Can you work these out from the model? Positions are in its coordinate system, mm. Face numbers are marked on the shaded views. A direction names the side the tool comes from. Coordinates: 2 decimals unless noted, no trailing zeros. Order: outer loops, then holes, each group sorted by start corner. A loop starts at its lowest first (then second) coordinate and runs counter-clockwise, first axis right, second up. Notation, with made-up numbers: (27.25, -7.75) -> (44.25, -7.75) arc R23 ccw to (44.25, 1.25) -> close; hole circle Ø6 at (56, 7.25). An arc over 180 degrees is marked (long way). Answer in a Markdown table with one row per item. Add a question column.
1. Imagine slicing it at D-D on y = -4.25. Write out the boundary of the cut face in (x, z), plus the area to 3 significant figures.
2. We'd pull the mould along Y, two halves only. Please class the marked faces 1, 2 and 3: pulls with the +Y half, pulls with the -Y half, needs draft (parallel to the pull), parting line crosses it, or undercut.
3. Will these pins go through, and if not, where does the flat tip stop? pin 1 (5 mm diameter, centred on y = -6.5, z = -10.5, fed in from +X); pin 2 (11 mm diameter, centred on y = -1, z = -21.5, fed in from +X); pin 3 (3 mm diameter, centred on y = -2.5, z = -21, fed in from -X); pin 4 (3 mm diameter, centred on x = 6.5, y = 7, fed in from +Z).
4. Imagine slicing it at B-B on x = 0. Write out the boundary of the cut face in (y, z) (1 decimal).
5. Imagine slicing it at A-A on y = 0. Write out the boundary of the cut face in (x, z) (3 decimals), plus the area to 3 significant figures.
6. If I drill on line 1 along Y through (x, z) = (0.25, -11.5); line 2 along Z through (x, y) = (6.75, 4.25); line 3 along Z through (x, y) = (-7.25, -0.5), over which ranges is the centre line in solid material (lowest first)? Write a range as [from, to].
7. Imagine slicing it at C-C on z = -22. Write out the boundary of the cut face in (x, y).
8. On a 3-axis mill with a long thin cutter (end or side, diameter ignored), from which of +Z, -Z, +X, -X, +Y, -Y can I reach the whole of each face in a straight line? I mean the marked faces 4, 5 and 6. Say none if no direction works.
from build123d import *

# Parameters (mm, degrees)
SKETCH1_R               = 4.725
BOSS_EXTRUDE1_DEPTH     = 12
SKETCH2_R               = 3.46
BOSS_EXTRUDE2_DEPTH     = 15
SKETCH5_R               = 10
BOSS_EXTRUDE3_DEPTH     = 15
CUT_EXTRUDE1_DEPTH      = 5
CUT_EXTRUDE1_DEPTH_BACK = 15
SKETCH4_W               = 2
SKETCH4_H               = 12
CUT_EXTRUDE2_DEPTH      = 10
CUT_EXTRUDE3_REACH      = 35.956
SKETCH6_R               = 2


with BuildPart() as part:
    # Sketch1 → Boss-Extrude1 (new body)
    with BuildSketch(Plane.XY):
        Circle(SKETCH1_R)
    extrude(amount=-BOSS_EXTRUDE1_DEPTH)

    # Sketch2 → Boss-Extrude2 (add)
    with BuildSketch(Plane.XY):
        Circle(SKETCH2_R)
    extrude(amount=BOSS_EXTRUDE2_DEPTH)

    # Sketch5 → Boss-Extrude3 (add)
    with BuildSketch(Plane(origin=(0, 0, -12), x_dir=(-1, 0, 0), z_dir=(0, 0, -1))):
        Circle(SKETCH5_R)
    extrude(amount=BOSS_EXTRUDE3_DEPTH)

    # Sketch3 → Cut-Extrude1 (cut, two sides: drawn at the far end of the back side and taken through both)
    with BuildSketch(Plane(origin=(0, 0, 0), x_dir=(0, 0, -1), z_dir=(1, 0, 0)).offset(-CUT_EXTRUDE1_DEPTH_BACK)):
        Polygon((27, -5), (27, 5), (17, 7.679491924), (17, -7.679491924), align=None)
    extrude(amount=CUT_EXTRUDE1_DEPTH + CUT_EXTRUDE1_DEPTH_BACK, mode=Mode.SUBTRACT)

    # Sketch4 → Cut-Extrude2 (cut)
    with BuildSketch(Plane(origin=(0, 0, -27), x_dir=(-1, 0, 0), z_dir=(0, 0, -1))):
        with Locations((-9, 0)):
            Rectangle(SKETCH4_W, SKETCH4_H)
    extrude(amount=-CUT_EXTRUDE2_DEPTH, mode=Mode.SUBTRACT)

    # Sketch6 → Cut-Extrude3 (cut, up to next)
    with BuildSketch(Plane(origin=(8, 0, 0), x_dir=(0, 0, -1), z_dir=(1, 0, 0)), mode=Mode.PRIVATE) as cut_extrude3_sk1:
        with Locations((22, 0)):
            Circle(SKETCH6_R)
    cut_extrude3_tool1 = extrude(cut_extrude3_sk1.sketch, amount=-CUT_EXTRUDE3_REACH, mode=Mode.PRIVATE) & part.part
    add(cut_extrude3_tool1.solids().sort_by_distance((8, 0, -22))[0], mode=Mode.SUBTRACT)


solid = part.part
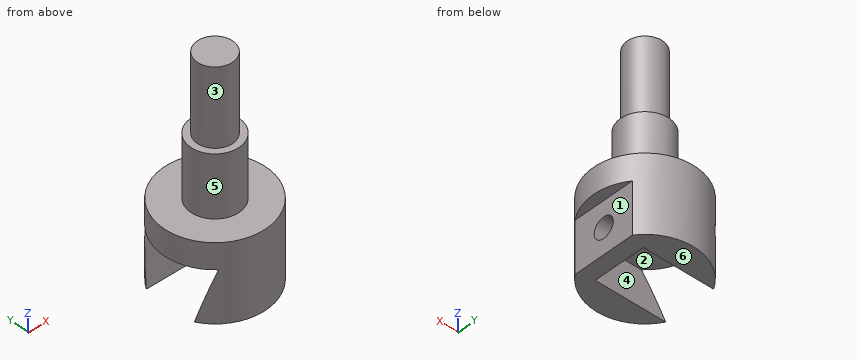
Answers follow:
| question | item | result |
|---|---|---|
| 1 | outline | (-9.05, -17) -> (5, -17) -> (5, -27) -> (8, -27) -> (8, -17) -> (9.05, -17) -> (9.05, -12) -> (2.06, -12) -> (2.06, 0) -> (-2.06, 0) -> (-2.06, -12) -> (-9.05, -12) -> close |
| 1 | area | 170 mm² |
| 2 | face 1 | needs draft |
| 2 | face 2 | undercut |
| 2 | face 3 | parting line crosses it |
| 3 | pin 1 | stops at x = 8.93 |
| 3 | pin 2 | stops at x = 10 |
| 3 | pin 3 | stops at x = 5 |
| 3 | pin 4 | stops at z = -12 |
| 4 | outline | (-10, -27) -> (-5, -27) -> (-7.7, -17) -> (7.7, -17) -> (5, -27) -> (10, -27) -> (10, -12) -> (4.7, -12) -> (4.7, 0) -> (3.5, 0) -> (3.5, 15) -> (-3.5, 15) -> (-3.5, 0) -> (-4.7, 0) -> (-4.7, -12) -> (-10, -12) -> close |
| 5 | outline | (-10, -17) -> (5, -17) -> (5, -20) -> (8, -20) -> (8, -17) -> (10, -17) -> (10, -12) -> (4.725, -12) -> (4.725, 0) -> (3.46, 0) -> (3.46, 15) -> (-3.46, 15) -> (-3.46, 0) -> (-4.725, 0) -> (-4.725, -12) -> (-10, -12) -> close; (5, -27) -> (8, -27) -> (8, -24) -> (5, -24) -> close |
| 5 | area | 335 mm² |
| 6 | line 1 | y = [-4.72, 4.72] |
| 6 | line 2 | z = [-27, -12] |
| 6 | line 3 | z = [-17, -12] |
| 7 | outline | (-7.73, -6.34) arc R10 ccw to (8, -6) -> (8, -2) -> (5, -2) -> (5, -6.34) -> close; (-7.73, 6.34) -> (5, 6.34) -> (5, 2) -> (8, 2) -> (8, 6) arc R10 ccw to start |
| 8 | face 4 | -X |
| 8 | face 5 | +Z |
| 8 | face 6 | -Z, +X, -X, +Y, -Y |
